Here's how the part is built. I have some questions about the finished solid (model axes, mm). A direction names the side the tool comes from. Round coordinates to 2 decimals unless told otherwise and drop trailing zeros. Write each loop counter-clockwise with the first axis right and the second up, starting at its lowest first coordinate (ties: lowest second). Pieces come first, ordered by that corner, then holes. Notation, with made-up numbers: (40, 13.5) -> (69, 13.5) arc R17 cw to (69, 21.5) -> close; hole circle Ø6 at (75.25, 27.25). An arc over 180 degrees is marked (long way). Put each result on its own line as item: value. Start each with the question number.
1) I want a section at B-B, the plane z = 26.75. Give the number of separate pieces and of enclosed holes in the cut face, then the cut area to 3 significant figures.
2) Which directions (+Z, -Z, +X, -X, +Y, -Y) give clear straight access to the entire face, cutting with the end or side of a thin tool? Please do faces 1 (the cylindrical face through (83.1, 12.5, 17)), 2 (the flat face through (79.1, -7.4, 32)), 3 (the flat face through (83, 18.93, 15)), 4 (the flat face through (61.338, 21.972, 19.296)).
3) If I drill on line 1 along Y through (x, z) = (83, 17.3); line 2 along X through (y, z) = (15.5, 16.7); line 3 along Y through (x, z) = (69, 24.5), over which ranges is the centre line in solid material (lowest first)? Write a range as [from, to].
4) I want a section at D-D, the plane x = 78.5. List the corners of the cut face in (y, z) for me.
5) We'd pull the mould along Y, two halves only. Please class faces 5 (the flat face through (49, 21, 32)), 6 (the flat face through (62, 0, 31)), 7 (the flat face through (74.533, -11.316, 31.986)): released by +Y, released by -Y, zero draft, split by the parting line, or undercut.
6) I want a section at A-A, the plane x = 46.5. List the corners of the cut face in (y, z) for me.
7) Will these pins go through, and if not, where does the flat tip stop? P1, Ø1.6, axis at y = -21, z = 15, coming from the -X side; P2, Ø8, axis at x = 59.5, y = -5, coming from the -Z side.
8) I want a section at C-C, the plane z = 17. List the corners of the cut face in (x, y) for me.
from build123d import *

# Parameters (mm, degrees)
SKETCH105_R                     = 4.3
SKETCH105_R_2                   = 2.85
PAD057_DEPTH                    = 2
SKETCH106_W                     = 6
SKETCH106_H                     = 6
PAD058_DEPTH                    = 17
SKETCH107_R                     = 1.7
PAD059_DEPTH                    = 2
SKETCH107_LINEARPATTERN002_2_R  = 1.7
PAD059_LINEARPATTERN002_2_DEPTH = 2
SKETCH106_LINEARPATTERN002_2_W  = 6
SKETCH106_LINEARPATTERN002_2_H  = 6
PAD058_LINEARPATTERN002_2_DEPTH = 17
PAD060_DEPTH                    = 6


with BuildPart() as part:
    # Sketch105 → Pad057 (new body)
    with BuildSketch(Plane.XY):
        with BuildLine():
            Line((3.464102, 6), (21, 6))
            Line((22.716302, 6), (21, 6))
            Line((22.716302, 6), (33.500258, 16.783955))
            Line((33.500258, 16.783955), (33.500258, 24.930573))
            Line((33.500258, 24.930573), (39.500258, 24.930573))
            Line((39.500258, 24.930573), (39.500258, 15.5))
            ThreePointArc((38.650792, 13.449208), (39.279489, 14.390119), (39.500258, 15.5))
            Line((26.786802, 1.585219), (38.650792, 13.449208))
            ThreePointArc((26.786802, -1.585219), (27, 0), (26.786802, 1.585219))
            Line((26.786802, -1.585219), (38.650792, -13.449208))
            ThreePointArc((39.500258, -15.5), (39.279489, -14.390119), (38.650792, -13.449208))
            Line((39.500258, -24.930573), (39.500258, -15.5))
            Line((33.500258, -24.930573), (39.500258, -24.930573))
            Line((33.500258, -16.783955), (33.500258, -24.930573))
            Line((22.716302, -6), (33.500258, -16.783955))
            Line((21, -6), (22.716302, -6))
            Line((3.464102, -6), (21, -6))
            Line((3.464102, -6), (8.111697, -14.049871))
            ThreePointArc((8.500258, -15.5), (8.401434, -14.749358), (8.111697, -14.049871))
            Line((8.500258, -24.930573), (8.500258, -15.5))
            Line((2.500258, -24.930573), (8.500258, -24.930573))
            Line((2.500258, -16.330573), (2.500258, -24.930573))
            Line((-5.196152, -3), (2.500258, -16.330573))
            ThreePointArc((-5.196152, 3), (-6, 0), (-5.196152, -3))
            Line((-5.196152, 3), (2.500258, 16.330573))
            Line((2.500258, 16.330573), (2.500258, 24.930573))
            Line((2.500258, 24.930573), (8.500258, 24.930573))
            Line((8.500258, 24.930573), (8.500258, 15.5))
            ThreePointArc((8.111697, 14.049871), (8.401434, 14.749358), (8.500258, 15.5))
            Line((3.464102, 6), (8.111697, 14.049871))
        make_face()
        Circle(SKETCH105_R, mode=Mode.SUBTRACT)
        with Locations((21, 0)):
            Circle(SKETCH105_R_2, mode=Mode.SUBTRACT)
    extrude(amount=PAD057_DEPTH)

    # Sketch106 (on Face33 of Pad057) → Pad058 (join)
    with BuildSketch(Plane(origin=(0, 0, 0), x_dir=(1, 0, 0), z_dir=(0, 0, -1))):
        with Locations((5.5, 21.93)):
            Rectangle(SKETCH106_W, SKETCH106_H)
    pad058 = extrude(amount=PAD058_DEPTH)

    # Sketch107 → Pad059 (join)
    with BuildSketch(Plane.XY.offset(-15)):
        with BuildLine():
            Line((2.5, -18.93), (2.5, -15.5))
            ThreePointArc((8.5, -15.5), (5.5, -12.5), (2.5, -15.5))
            Line((8.5, -18.93), (8.5, -15.5))
            Line((2.5, -18.93), (8.5, -18.93))
        make_face()
        with Locations((5.5, -15.5)):
            Circle(SKETCH107_R, mode=Mode.SUBTRACT)
    pad059 = extrude(amount=PAD059_DEPTH)

    # Sketch107 LinearPattern002 2 → Pad059 LinearPattern002 2 (add)
    with BuildSketch(Plane(origin=(31, 0, -15), x_dir=(1, 0, 0), z_dir=(0, 0, 1))):
        with BuildLine():
            Line((2.5, -18.93), (2.5, -15.5))
            ThreePointArc((8.5, -15.5), (5.5, -12.5), (2.5, -15.5))
            Line((8.5, -18.93), (8.5, -15.5))
            Line((2.5, -18.93), (8.5, -18.93))
        make_face()
        with Locations((5.5, -15.5)):
            Circle(SKETCH107_LINEARPATTERN002_2_R, mode=Mode.SUBTRACT)
    pad059_linearpattern002_2 = extrude(amount=PAD059_LINEARPATTERN002_2_DEPTH)

    # Sketch106 LinearPattern002 2 → Pad058 LinearPattern002 2 (add)
    with BuildSketch(Plane(origin=(31, 0, 0), x_dir=(1, 0, 0), z_dir=(0, 0, -1))):
        with Locations((5.5, 21.93)):
            Rectangle(SKETCH106_LINEARPATTERN002_2_W, SKETCH106_LINEARPATTERN002_2_H)
    pad058_linearpattern002_2 = extrude(amount=PAD058_LINEARPATTERN002_2_DEPTH)

    # Mirrored003: Pad059, Pad058, Pad059 LinearPattern002 2, Pad058 LinearPattern002 2 across Sketch107 H_Axis
    add(pad059.mirror(Plane(origin=(0, 0, -15), x_dir=(0, 0, 1), z_dir=(0, 1, 0))))
    add(pad058.mirror(Plane(origin=(0, 0, -15), x_dir=(0, 0, 1), z_dir=(0, 1, 0))))
    add(pad059_linearpattern002_2.mirror(Plane(origin=(0, 0, -15), x_dir=(0, 0, 1), z_dir=(0, 1, 0))))
    add(pad058_linearpattern002_2.mirror(Plane(origin=(0, 0, -15), x_dir=(0, 0, 1), z_dir=(0, 1, 0))))

    # Sketch108 (on Face36 of MultiTransform003) → Pad060 (join)
    with BuildSketch(Plane.XZ.offset(24.93)):
        Polygon((8.5, 0), (21, -6.5), (33.5, 0), (33.5, -2), (22.923077, -7.5), (33.5, -13), (33.5, -15), (21, -8.5), (8.5, -15), (8.5, -13), (19.076923, -7.5), (8.5, -2), align=None)
    pad060 = extrude(amount=-PAD060_DEPTH)

    # Mirrored004: Pad060 across XZ
    add(pad060.mirror(Plane.XZ))


with BuildPart() as part_1:
    # Body028 placement: moved
    add(part.part.moved(Location((46.5, 0, 31))))


solid = part_1.part
Findings:
1. separate pieces: 8
1. enclosed holes: 0
1. area: 236 mm2
2. face 1: -Z
2. face 2: +Z, -Z, +X
2. face 3: -Z, +X, -X
2. face 4: -Z, +Y, -Y
3. line 1: y = [-24.93, -17.2], [-13.8, -12.5], [12.5, 13.8], [17.2, 24.93]
3. line 2: x = [49, 50.3], [53.7, 55], [80, 81.3], [84.7, 86]
3. line 3: y = [-24.93, -18.93], [18.93, 24.93]
4. outline: (-24.93, 16.78) -> (-18.93, 16.78) -> (-18.93, 18.78) -> (-24.93, 18.78) -> close; (-24.93, 28.22) -> (-18.93, 28.22) -> (-18.93, 30.22) -> (-24.93, 30.22) -> close; (-15.28, 31) -> (-6.8, 31) -> (-6.8, 33) -> (-15.28, 33) -> close; (6.8, 31) -> (15.28, 31) -> (15.28, 33) -> (6.8, 33) -> close; (18.93, 16.78) -> (24.93, 16.78) -> (24.93, 18.78) -> (18.93, 18.78) -> close; (18.93, 28.22) -> (24.93, 28.22) -> (24.93, 30.22) -> (18.93, 30.22) -> close
5. face 5: zero draft
5. face 6: undercut
5. face 7: released by -Y
6. outline: (-12, 31) -> (-4.3, 31) -> (-4.3, 33) -> (-12, 33) -> close; (4.3, 31) -> (12, 31) -> (12, 33) -> (4.3, 33) -> close
7. P1: stops at x = 49
7. P2: stops at z = 31
8. outline: (49, -24.93) -> (56.92, -24.93) -> (56.92, -18.93) -> (55, -18.93) -> (55, -15.5) arc R3 ccw to (49, -15.5) -> close; (49, 15.5) arc R3 ccw to (55, 15.5) -> (55, 18.93) -> (56.92, 18.93) -> (56.92, 24.93) -> (49, 24.93) -> close; (78.08, -24.93) -> (86, -24.93) -> (86, -15.5) arc R3 ccw to (80, -15.5) -> (80, -18.93) -> (78.08, -18.93) -> close; (78.08, 18.93) -> (80, 18.93) -> (80, 15.5) arc R3 ccw to (86, 15.5) -> (86, 24.93) -> (78.08, 24.93) -> close; hole circle Ø3.4 at (52, -15.5); hole circle Ø3.4 at (52, 15.5); hole circle Ø3.4 at (83, -15.5); hole circle Ø3.4 at (83, 15.5)
